Autodesk Inventor part; units mm, degrees
ref_plane "YZ Plane" through (0, 0, 0) normal (1, 0, 0) x (0, 1, 0)
ref_plane "XZ Plane" through (0, 0, 0) normal (0, 1, 0) x (-1, 0, 0)
ref_plane "XY Plane" through (0, 0, 0) normal (0, 0, 1) x (1, 0, 0)
sketch "Sketch1" plane through (0, 0, 0) normal (0, 1, 0) x (-1, 0, 0)
  line L0 (0, -2.6558) -> (-2.3, -1.3279)
  line L1 (-2.3, -1.3279) -> (-2.3, 1.3279)
  line L2 (-2.3, 1.3279) -> (0, 2.6558)
  line L3 (0, 2.6558) -> (2.3, 1.3279)
  line L4 (2.3, 1.3279) -> (2.3, -1.3279)
  line L5 (2.3, -1.3279) -> (0, -2.6558)
  point P0 (0, 0)
  point P1 (0, 0)
  dimension "d0" = 4.6
extrude "Extrusion1" add sketch "Sketch1" along normal blind 28
sketch "Sketch2" plane through (0, 28, 0) normal (0, 1, 0) x (1, 0, 0)
  circle A0 centre (0, 0) radius 1.5
  dimension "d3" = 3
extrude "Extrusion2" cut sketch "Sketch2" against normal blind 15
sketch "Sketch3" plane through (0, 0, 0) normal (0, -1, 0) x (1, 0, 0)
  circle A0 centre (0, 0) radius 1.5
  dimension "d6" = 3
extrude "Extrusion3" add sketch "Sketch3" along normal blind 6
properties part number "M3_28_MM_STANDOFF_PIN"
Geometry: final body of the model. Coordinates: model frame, mm. A direction names the side the tool comes from. Give positions to 0.01 mm unless a question says otherwise; leave off trailing zeros. Loops run counter-clockwise (first coordinate to the right, second up) from the corner with the lowest first, then second, coordinate; pieces in that order, holes last. Notation, with made-up numbers: (5.5, -18.75) - (19.5, -18.75) arc R19 ccw to (19.5, -8.75) - close; hole circle Ø11 at (8, 81). An arc over 180 degrees is marked (long way). Answer as CSV lines item,"result". Start each with the question number.
1. Draft query along Z for faces 4 (the face through (2, 28, 0)), 5 (the face through (-1.5, 20.6, -0.07)), 6 (the face through (1.17, 13.8, 1.98)). Return one class per face: released by +Z, released by -Z, zero draft, split by the parting line, or undercut.
2. Reachability of faces 1 (the face through (2, 0, 0)), 2 (the face through (2.3, 14, 0)), 3 (the face through (0, 13, 0)) from +Z, -Z, +X, -X, +Y, -Y: full face, straight path, thin tool, end or side. Return the list, or none.
3. Ray query, L1, parallel to X at y = 21.5, z = 0; L2, parallel to X at y = 19, z = 0.65; L3, parallel to Y at x = 2, z = -1.2. Return the intervals inside material, ascending.
4. Section A-A, the plane y = 16. Return loops of the section in (x, z).
5. Section D-D, the plane z = -2.15. Return loops of the section in (x, y).
6. Section B-B, the plane z = 0. Return loops of the section in (x, y), plus the area to 3 significant figures.
7. Section C-C, the plane x = 0.7. Return loops of the section in (y, z), plus the area to 3 significant figures.
Answers:
1,face 4,"zero draft"
1,face 5,"undercut"
1,face 6,"released by +Z"
2,face 1,"-Y"
2,face 2,"+Z, -Z, +X, +Y, -Y"
2,face 3,"+Y"
3,L1,"x = -2.3 to -1.5, 1.5 to 2.3"
3,L2,"x = -2.3 to -1.35, 1.35 to 2.3"
3,L3,"y = 0 to 28"
4,outline,"(-2.3, -1.33) - (0, -2.66) - (2.3, -1.33) - (2.3, 1.33) - (0, 2.66) - (-2.3, 1.33) - close; hole circle Ø3 at (0, 0)"
5,outline,"(-0.88, 0) - (0.88, 0) - (0.88, 28) - (-0.88, 28) - close"
6,outline,"(-2.3, 0) - (-1.5, 0) - (-1.5, -6) - (1.5, -6) - (1.5, 0) - (2.3, 0) - (2.3, 28) - (1.5, 28) - (1.5, 13) - (-1.5, 13) - (-1.5, 28) - (-2.3, 28) - close"
6,area,"102 mm2"
7,outline,"(-6, -1.33) - (0, -1.33) - (0, -2.25) - (28, -2.25) - (28, -1.33) - (13, -1.33) - (13, 1.33) - (28, 1.33) - (28, 2.25) - (0, 2.25) - (0, 1.33) - (-6, 1.33) - close"
7,area,"102 mm2"
